```python
from build123d import *

# Parameters (mm, degrees)
BOSS_EXTRU_1_DEPTH       = 60
ESQUISSE2_R              = 2.85
ENL_V_MAT_EXTRU_1_DEPTH  = 30
ESQUISSE3_R              = 2.85
ENL_V_MAT_EXTRU_2_DEPTH  = 1.2
ENL_V_START              = -1.2
ESQUISSE4_R              = 5.5
ENL_V_MAT_EXTRU_3_DEPTH  = 30
CHANFREIN1_SIZE          = 5
CHANFREIN3_SIZE          = 10
ENL_V_MAT_EXTRU_5_REACH  = 83.872
ESQUISSE7_R              = 5.5
CHANFREIN4_SIZE          = 2
CHANFREIN4_SIZE2         = 7.464101615
BOSS_EXTRU_3_DEPTH       = 60
ESQUISSE10_R             = 2
ENL_V_MAT_EXTRU_7_DEPTH  = 60
ESQUISSE11_R             = 4
ENL_V_MAT_EXTRU_8_DEPTH  = 3
CHANFREIN5_SIZE          = 8
ESQUISSE12_W             = 5
ESQUISSE12_H             = 15
ENL_V_MAT_EXTRU_9_DEPTH  = 84.554960758
ESQUISSE13_W             = 15
ESQUISSE13_H             = 18
ENL_V_MAT_EXTRU_10_DEPTH = 84.554960758


with BuildPart() as part:
    # Esquisse1 → Boss.-Extru.1 (new body)
    with BuildSketch(Plane.XY):
        Polygon((0, 0), (44.894653535, 0), (41.742346142, 11.764571353), (12.764571353, 4), (5, 32.977774789), (0, 32.977774789), align=None)
    extrude(amount=BOSS_EXTRU_1_DEPTH)

    # Esquisse2 → Enlèv. mat.-Extru.1 (cut)
    with BuildSketch(Plane(origin=(12.909507207, 3.459092031, 0), x_dir=(0, 0, -1), z_dir=(0.965925826289071, 0.258819045102511, 0))):
        with Locations(Location((-51, 23.559989136, 0), (0, 0, 90))):
            Circle(ESQUISSE2_R)
        with Locations(Location((-9, 23.559989136, 0), (0, 0, 90))):
            Circle(ESQUISSE2_R)
    extrude(amount=-ENL_V_MAT_EXTRU_1_DEPTH, mode=Mode.SUBTRACT)

    # Esquisse3 → Enlèv. mat.-Extru.2 (cut)
    with BuildSketch(Plane(origin=(-0.144935854, 0.540907969, 0), x_dir=(0.96592582628907, 0.2588190451025147, 0), z_dir=(-0.25881904510251463, 0.9659258262890699, 0))):
        with Locations(Location((32.364905312, -9, 0), (0, 0, 180))):
            Circle(ESQUISSE3_R)
        with Locations(Location((32.364905312, -51, 0), (0, 0, 180))):
            Circle(ESQUISSE3_R)
    extrude(amount=-ENL_V_MAT_EXTRU_2_DEPTH, mode=Mode.SUBTRACT)

    # Esquisse4 → Enlèv. mat.-Extru.3 (cut)
    with BuildSketch(Plane(origin=(12.909507207, 3.459092031, 0), x_dir=(0, 0, -1), z_dir=(0.965925826289071, 0.258819045102511, 0)).offset(ENL_V_START)):
        with Locations(Location((-51, 23.559989136, 0), (0, 0, 90))):
            Circle(ESQUISSE4_R)
        with Locations(Location((-9, 23.559989136, 0), (0, 0, 90))):
            Circle(ESQUISSE4_R)
    extrude(amount=-ENL_V_MAT_EXTRU_3_DEPTH, mode=Mode.SUBTRACT)

    # Chanfrein1
    chanfrein1_edges = [part.edges().sort_by_distance(p)[0] for p in [
        (12.764571353, 4, 30),
    ]]
    chamfer(chanfrein1_edges, length=CHANFREIN1_SIZE)

    # Chanfrein3
    chanfrein3_edges = [part.edges().sort_by_distance(p)[0] for p in [
        (0, 0, 30),
    ]]
    chamfer(chanfrein3_edges, length=CHANFREIN3_SIZE)

    # Enlèv. mat.-Extru.5: up to this plane
    enl_v_mat_extru_5_end = Plane(origin=(31.427744907, 7.758450865, 51), z_dir=(-0.2588190451025147, 0.96592582628907, 0))
    # Esquisse7 → Enlèv. mat.-Extru.5 (cut, up to the surface)
    with BuildSketch(Plane.XZ, mode=Mode.PRIVATE) as enl_v_mat_extru_5_sk1:
        with Locations((31.117162053, 51)):
            Circle(ESQUISSE7_R)
    enl_v_mat_extru_5_tool1 = split(extrude(enl_v_mat_extru_5_sk1.sketch, amount=-ENL_V_MAT_EXTRU_5_REACH, mode=Mode.PRIVATE), bisect_by=enl_v_mat_extru_5_end, keep=Keep.BOTH, mode=Mode.PRIVATE)
    add(enl_v_mat_extru_5_tool1.solids().sort_by_distance((31.117162, 0, 51))[0], mode=Mode.SUBTRACT)
    # Esquisse7 → Enlèv. mat.-Extru.5 (cut, up to the surface)
    with BuildSketch(Plane.XZ, mode=Mode.PRIVATE) as enl_v_mat_extru_5_sk2:
        with Locations((31.117162053, 9)):
            Circle(ESQUISSE7_R)
    enl_v_mat_extru_5_tool2 = split(extrude(enl_v_mat_extru_5_sk2.sketch, amount=-ENL_V_MAT_EXTRU_5_REACH, mode=Mode.PRIVATE), bisect_by=enl_v_mat_extru_5_end, keep=Keep.BOTH, mode=Mode.PRIVATE)
    add(enl_v_mat_extru_5_tool2.solids().sort_by_distance((31.117162, 0, 9))[0], mode=Mode.SUBTRACT)

    # Chanfrein4
    chanfrein4_edges = [part.edges().sort_by_distance(p)[0] for p in [
        (41.742346142, 11.764571353, 30),
    ]]
    chanfrein4_side = [part.faces().sort_by_distance(p)[0] for p in [
        (43.318499838, 5.882285677, 30),
    ]]
    chamfer(chanfrein4_edges, length=CHANFREIN4_SIZE, length2=CHANFREIN4_SIZE2, reference=chanfrein4_side[0])

    # Esquisse8 → Boss.-Extru.3 (add)
    with BuildSketch(Plane.XY.offset(60)):
        Polygon((42.259984232, 9.8327197), (47.894653535, 9.8327197), (47.894653535, 0), (44.894653535, 0), align=None)
    extrude(amount=-BOSS_EXTRU_3_DEPTH)

    # Esquisse10 → Enlèv. mat.-Extru.7 (cut)
    with BuildSketch(Plane(origin=(0, 9.8327197, 0), x_dir=(1, 0, 0), z_dir=(0, 1, 0))):
        with Locations(Location((40.75, -14.5, 0), (0, 0, 180))):
            Circle(ESQUISSE10_R)
        with Locations(Location((40.75, -45.5, 0), (0, 0, 180))):
            Circle(ESQUISSE10_R)
    extrude(amount=-ENL_V_MAT_EXTRU_7_DEPTH, mode=Mode.SUBTRACT)

    # Esquisse11 → Enlèv. mat.-Extru.8 (cut)
    with BuildSketch(Plane(origin=(0, 9.8327197, 0), x_dir=(1, 0, 0), z_dir=(0, 1, 0))):
        with Locations(Location((40.75, -14.5, 0), (0, 0, 180))):
            Circle(ESQUISSE11_R)
        with Locations(Location((40.75, -45.5, 0), (0, 0, 180))):
            Circle(ESQUISSE11_R)
    extrude(amount=-ENL_V_MAT_EXTRU_8_DEPTH, mode=Mode.SUBTRACT)

    # Chanfrein5
    chanfrein5_edges = [part.edges().sort_by_distance(p)[0] for p in [
        (47.894653535, 4.91635985, 0),
        (47.894653535, 4.91635985, 60),
    ]]
    chamfer(chanfrein5_edges, length=CHANFREIN5_SIZE)

    # Esquisse12 → Enlèv. mat.-Extru.9 (cut, through all)
    with BuildSketch(Plane.XZ):
        with Locations((17.5, 30)):
            Rectangle(ESQUISSE12_W, ESQUISSE12_H)
        with Locations((27.5, 30)):
            Rectangle(ESQUISSE12_W, ESQUISSE12_H)
    extrude(amount=-ENL_V_MAT_EXTRU_9_DEPTH, mode=Mode.SUBTRACT)

    # Esquisse13 → Enlèv. mat.-Extru.10 (cut, through all)
    with BuildSketch(Plane.ZY):
        with Locations((30, 19.977774789)):
            Rectangle(ESQUISSE13_W, ESQUISSE13_H)
    extrude(amount=-ENL_V_MAT_EXTRU_10_DEPTH, mode=Mode.SUBTRACT)


solid = part.part
```
Source: CAD feature listing. Evaluate the final solid. Frame: model axes, mm. A direction names the side the tool comes from. Coordinates: 2 decimals unless noted, no trailing zeros. Write each loop counter-clockwise with the first axis right and the second up, starting at its lowest first coordinate (ties: lowest second). Pieces come first, ordered by that corner, then holes. Notation, with made-up numbers: (-20.75, 48.5) -> (-0.75, 48.5) arc R30 cw to (-0.75, 72.5) -> close; hole circle Ø7 at (4, -24). An arc over 180 degrees is marked (long way). Return JSON: item names as keys, results as strings. Group by question number.
1) Section query C-C, the plane z = 39.5. Return loops of the section in (x, y).
2) Mould query, pull axis X, two halves, no side actions, for faces 5 (the face through (5, 5, 30)), 6 (the face through (3, 32.978, 30)), 7 (the face through (31.87, 8.51, 48.22)). Classes: +X half, -X half, draft (parallel to the pull), parting line (faces both ways), or undercut.
3) Ray query, line 1 along Z through (x, y) = (5, 15.5); line 2 along Z through (x, y) = (3, 27); line 3 along Z through (x, y) = (40.75, 8.25). Return the intervals inside material, ascending.
4) Section query A-A, the plane z = 23.5. Return loops of the section in (x, y).
5) Section query B-B, the plane y = 17. Return loops of the section in (x, z).
6) Contact query for flat-ended pins moving along their axis: P1, Ø3.5, axis at x = 40.75, z = 14.5, coming from the -Y side; P2, Ø8, axis at x = 7.5, z = 12, coming from the -Y side; P3, Ø1.5, axis at y = 22.5, z = 10.5, coming from the +X side; P4, Ø12, axis at y = 20.5, z = 38.5, coming from the +X side. Output: stop coordinate, or through.
7) Set-up query: faces 1 (the face through (5, 10.978, 30)), 2 (the face through (28.6, 7, 10.1)), 3 (the face through (43.924, 8.354, 43.066)), 4 (the face through (5.04, 28.19, 48.63)). Return all of +Z, -Z, +X, -X, +Y, -Y with unobstructed straight access to the full face (end or side cutting, diameter ignored); none if empty.
8) Section query D-D, the plane z = 51. Return loops of the section in (x, y), plus the area to 3 significant figures.
From the geometry:
{
 "1": {"outline": "(0, 10) -> (10, 0) -> (47.89, 0) -> (47.89, 9.83) -> (34.53, 9.83) -> (17.59, 5.29) -> (11.47, 8.83) -> (5, 32.98) -> (0, 32.98) -> close"},
 "2": {"face 5": "-X half", "face 6": "draft", "face 7": "undercut"},
 "3": {"line 1": "0 to 22.5, 37.5 to 60", "line 2": "0 to 3.78, 14.22 to 22.5, 37.5 to 45.78, 56.22 to 60", "line 3": "0.86 to 10.5, 18.5 to 41.5, 49.5 to 59.14"},
 "4": {"outline": "(0, 10) -> (10, 0) -> (15, 0) -> (15, 6.79) -> (11.47, 8.83) -> (10.89, 10.98) -> (0, 10.98) -> close; (0, 28.98) -> (6.07, 28.98) -> (5, 32.98) -> (0, 32.98) -> close; (20, 0) -> (25, 0) -> (25, 7.28) -> (20, 5.94) -> close; (30, 0) -> (47.89, 0) -> (47.89, 9.83) -> (34.53, 9.83) -> (30, 8.62) -> close"},
 "5": {"outline": "(0, 0) -> (9.28, 0) -> (9.28, 22.5) -> (0, 22.5) -> close; (0, 37.5) -> (9.28, 37.5) -> (9.28, 60) -> (0, 60) -> close"},
 "6": {"P1": "through", "P2": "y = 0", "P3": "x = 8.01", "P4": "x = 9.95"},
 "7": {"face 1": "+X, -X", "face 2": "-Y", "face 3": "+Y", "face 4": "none"},
 "8": {"outline": "(0, 10) -> (10, 0) -> (25.62, 0) -> (25.62, 6.2) -> (28.67, 7.02) -> (28.36, 8.18) -> (17.59, 5.29) -> (11.47, 8.83) -> (7.55, 23.46) -> (6.39, 23.15) -> (7.08, 20.59) -> (0, 18.7) -> close; (0, 30.09) -> (4.23, 31.22) -> (4.91, 28.66) -> (6.07, 28.97) -> (5, 32.98) -> (0, 32.98) -> close; (33.87, 9.66) -> (34.18, 8.5) -> (36.62, 9.15) -> (36.62, 0) -> (47.89, 0) -> (47.89, 9.83) -> (34.53, 9.83) -> close", "area": "390 mm²"}
}
